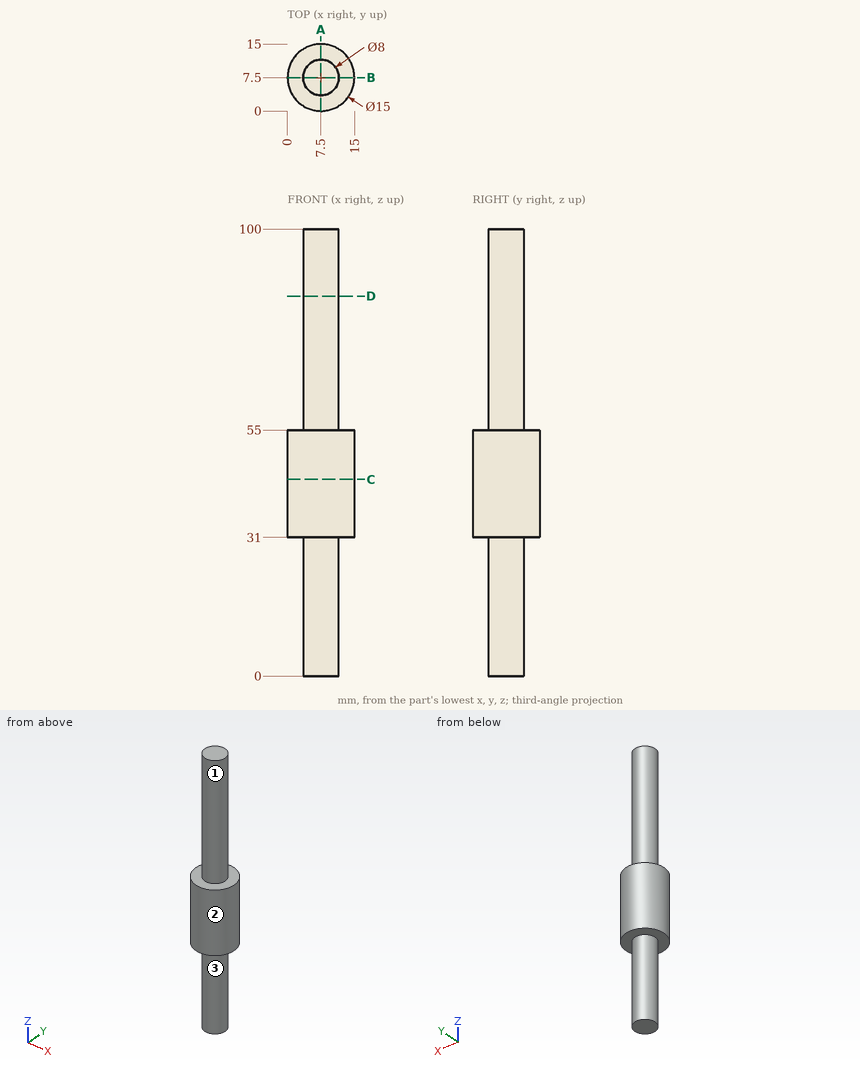
For this review, use the dimensioned drawing (mm, ordinates from the lowest corner) and the shaded views. A direction names the side the tool comes from. Coordinates: 2 decimals unless noted, no trailing zeros. Loops run counter-clockwise (first coordinate to the right, second up) from the corner with the lowest first, then second, coordinate; pieces in that order, holes last. Notation, with made-up numbers: (49, 69.25) - (64, 69.25) arc R24 cw to (64, 104.25) - close; hole circle Ø2 at (55.5, -31). An arc over 180 degrees is marked (long way). Use CSV: the item, a comma, the result in double quotes. Start each with the question number.
1) For pin 1 Ø6 at (y, z) = (8.5, 15) entering from +X; pin 2 Ø2 at (y, z) = (4.5, 27.5) entering from -X; pin 3 Ø6 at (x, z) = (12.5, 40) entering from +Y, all flat-tipped, find the tip position at first contact; note any pin that passes through.
2) Wall thickness on L1, parallel to Y at x = 7.5, z = 65; L2, parallel to Z at x = 13, y = 8.25; L3, parallel to Y at x = 8.5, z = 38.5: over which ranges is each line inside the solid? List them lowest first. Write a range as from..to.
3) Tool access review of the marked faces 1, 2 and 3: name each direction out of +Z, -Z, +X, -X, +Y, -Y from which nothing blocks a thin tool from reaching the whole face with its end or side.
4) Consider section D-D on z = 85. Write out the cut boundary in (x, y), then the cut area to 3 significant figures.
5) Consider section C-C on z = 44. Write out the cut boundary in (x, y).
6) Consider section A-A on x = 7.5. Write out the cut boundary in (y, z).
Geometry says:
1,pin 1,"x = 11.5"
1,pin 2,"x = 4.04"
1,pin 3,"y = 14.73"
2,L1,"3.5..11.5"
2,L2,"31..55"
2,L3,"0.07..14.93"
3,face 1,"+Z"
3,face 2,"+Z, -Z"
3,face 3,"-Z"
4,outline,"circle Ø8 at (7.5, 7.5)"
4,area,"50.3 mm^2"
5,outline,"circle Ø15 at (7.5, 7.5)"
6,outline,"(0, 31) - (3.5, 31) - (3.5, 0) - (11.5, 0) - (11.5, 31) - (15, 31) - (15, 55) - (11.5, 55) - (11.5, 100) - (3.5, 100) - (3.5, 55) - (0, 55) - close"
